Model file for the job. Use its own axes, mm. Give positions to 0.01 mm unless a question says otherwise; leave off trailing zeros. Write each loop counter-clockwise with the first axis right and the second up, starting at its lowest first coordinate (ties: lowest second). Pieces come first, ordered by that corner, then holes. Notation, with made-up numbers: M 64,-2 L 95,-2 A27 cw 95,32 Z; hole C -21.5,53 d9. An arc over 180 degrees is marked long. Answer as a JSON object with one key per item and string values. Group by question number.
```python
from build123d import *

# Parameters (mm, degrees)
BOSS_EXTRUDE1_DEPTH = 10
CUT_EXTRUDE1_REACH  = 12
SKETCH2_R           = 1.5
CUT_EXTRUDE2_REACH  = 12
SKETCH3_R           = 1.3
SKETCH3_R_2         = 7.5


with BuildPart() as part:
    # Sketch1 → Boss-Extrude1 (new body)
    with BuildSketch(Plane.XY):
        with BuildLine():
            Line((-21, 100), (-29.51790497, 5.356611447))
            ThreePointArc((-29.51790497, 5.356611447), (0, 30), (29.51790497, 5.356611447))
            Line((29.51790497, 5.356611447), (21, 100))
            Line((21, 100), (-21, 100))
        make_face()
        with BuildLine():
            Line((-29.51790497, 5.356611447), (-30, 0))
            ThreePointArc((-30, 0), (0, -30), (30, 0))
            Line((30, 0), (29.51790497, 5.356611447))
            ThreePointArc((29.51790497, 5.356611447), (0, 30), (-29.51790497, 5.356611447))
        make_face()
    extrude(amount=BOSS_EXTRUDE1_DEPTH)

    # Sketch2 → Cut-Extrude1 (cut, up to next)
    with BuildSketch(Plane(origin=(0, 0, 0), x_dir=(-1, 0, 0), z_dir=(0, 0, -1)), mode=Mode.PRIVATE) as cut_extrude1_sk1:
        with Locations((7, 92)):
            Circle(SKETCH2_R)
    cut_extrude1_tool1 = extrude(cut_extrude1_sk1.sketch, amount=-CUT_EXTRUDE1_REACH, mode=Mode.PRIVATE) & part.part
    add(cut_extrude1_tool1.solids().sort_by_distance((-7, 92, 0))[0], mode=Mode.SUBTRACT)
    # Sketch2 → Cut-Extrude1 (cut, up to next)
    with BuildSketch(Plane(origin=(0, 0, 0), x_dir=(-1, 0, 0), z_dir=(0, 0, -1)), mode=Mode.PRIVATE) as cut_extrude1_sk2:
        with Locations((7, 77)):
            Circle(SKETCH2_R)
    cut_extrude1_tool2 = extrude(cut_extrude1_sk2.sketch, amount=-CUT_EXTRUDE1_REACH, mode=Mode.PRIVATE) & part.part
    add(cut_extrude1_tool2.solids().sort_by_distance((-7, 77, 0))[0], mode=Mode.SUBTRACT)
    # Sketch2 → Cut-Extrude1 (cut, up to next)
    with BuildSketch(Plane(origin=(0, 0, 0), x_dir=(-1, 0, 0), z_dir=(0, 0, -1)), mode=Mode.PRIVATE) as cut_extrude1_sk3:
        with Locations((-7, 77)):
            Circle(SKETCH2_R)
    cut_extrude1_tool3 = extrude(cut_extrude1_sk3.sketch, amount=-CUT_EXTRUDE1_REACH, mode=Mode.PRIVATE) & part.part
    add(cut_extrude1_tool3.solids().sort_by_distance((7, 77, 0))[0], mode=Mode.SUBTRACT)
    # Sketch2 → Cut-Extrude1 (cut, up to next)
    with BuildSketch(Plane(origin=(0, 0, 0), x_dir=(-1, 0, 0), z_dir=(0, 0, -1)), mode=Mode.PRIVATE) as cut_extrude1_sk4:
        with Locations((-7, 92)):
            Circle(SKETCH2_R)
    cut_extrude1_tool4 = extrude(cut_extrude1_sk4.sketch, amount=-CUT_EXTRUDE1_REACH, mode=Mode.PRIVATE) & part.part
    add(cut_extrude1_tool4.solids().sort_by_distance((7, 92, 0))[0], mode=Mode.SUBTRACT)

    # Sketch3 → Cut-Extrude2 (cut, up to next)
    with BuildSketch(Plane(origin=(0, 0, 0), x_dir=(-1, 0, 0), z_dir=(0, 0, -1)), mode=Mode.PRIVATE) as cut_extrude2_sk1:
        with Locations((0, 13)):
            Circle(SKETCH3_R)
    cut_extrude2_tool1 = extrude(cut_extrude2_sk1.sketch, amount=-CUT_EXTRUDE2_REACH, mode=Mode.PRIVATE) & part.part
    add(cut_extrude2_tool1.solids().sort_by_distance((0, 13, 0))[0], mode=Mode.SUBTRACT)
    # Sketch3 → Cut-Extrude2 (cut, up to next)
    with BuildSketch(Plane(origin=(0, 0, 0), x_dir=(-1, 0, 0), z_dir=(0, 0, -1)), mode=Mode.PRIVATE) as cut_extrude2_sk2:
        with Locations((13, 0)):
            Circle(SKETCH3_R)
    cut_extrude2_tool2 = extrude(cut_extrude2_sk2.sketch, amount=-CUT_EXTRUDE2_REACH, mode=Mode.PRIVATE) & part.part
    add(cut_extrude2_tool2.solids().sort_by_distance((-13, 0, 0))[0], mode=Mode.SUBTRACT)
    # Sketch3 → Cut-Extrude2 (cut, up to next)
    with BuildSketch(Plane(origin=(0, 0, 0), x_dir=(-1, 0, 0), z_dir=(0, 0, -1)), mode=Mode.PRIVATE) as cut_extrude2_sk3:
        with Locations((0, -13)):
            Circle(SKETCH3_R)
    cut_extrude2_tool3 = extrude(cut_extrude2_sk3.sketch, amount=-CUT_EXTRUDE2_REACH, mode=Mode.PRIVATE) & part.part
    add(cut_extrude2_tool3.solids().sort_by_distance((0, -13, 0))[0], mode=Mode.SUBTRACT)
    # Sketch3 → Cut-Extrude2 (cut, up to next)
    with BuildSketch(Plane(origin=(0, 0, 0), x_dir=(-1, 0, 0), z_dir=(0, 0, -1)), mode=Mode.PRIVATE) as cut_extrude2_sk4:
        with Locations((-13, 0)):
            Circle(SKETCH3_R)
    cut_extrude2_tool4 = extrude(cut_extrude2_sk4.sketch, amount=-CUT_EXTRUDE2_REACH, mode=Mode.PRIVATE) & part.part
    add(cut_extrude2_tool4.solids().sort_by_distance((13, 0, 0))[0], mode=Mode.SUBTRACT)
    # Sketch3 → Cut-Extrude2 (cut, up to next)
    with BuildSketch(Plane(origin=(0, 0, 0), x_dir=(-1, 0, 0), z_dir=(0, 0, -1)), mode=Mode.PRIVATE) as cut_extrude2_sk5:
        Circle(SKETCH3_R_2)
    cut_extrude2_tool5 = extrude(cut_extrude2_sk5.sketch, amount=-CUT_EXTRUDE2_REACH, mode=Mode.PRIVATE) & part.part
    add(cut_extrude2_tool5.solids().sort_by_distance((0, 0, 0))[0], mode=Mode.SUBTRACT)


solid = part.part
```
Q1. Wall check: L1, parallel to Y at x = 0, z = 5.5; L2, parallel to X at y = 76, z = 1.75; L3, parallel to Y at x = -8, z = 6. Give the ranges that are in metal, low to high.
Q2. Slice it at C-C, the plane z = 7. Count the separate pieces of the cut face and the enclosed holes in it, then the cut area to 3 significant figures.
Q3. Slice it at D-D, the plane x = 13. Write the cut outline in (y, z), then the cut area to 3 significant figures.
Q4. Two-plate mould, pull along X, no slides. Class faces 1 (the cylindrical face through (-0.66, -29.993, 4.93)), 2 (the flat face through (0, 36, 0)), 3 (the cylindrical face through (0.17, -11.71, 4.93)): +X half, -X half, draft (parallel to the pull), parting line (faces both ways), or undercut.
Q5. Slice it at B-B, the plane x = 0. Write the cut outline in (y, z), then the cut area to 3 significant figures.
Q6. Drop flat-ended pins along their axis: P1, Ø4, axis at y = 82, z = 9, coming from the +X side; P2, Ø4, axis at x = 21.5, z = 2, coming from the -Y side; P3, Ø5, axis at y = 55, z = 2.5, coming from the -X side (3 decimals). Give the stop position or say it passes through.
Q7. Slice it at A-A, the plane y = 92. Write the cut outline in (x, z).
Solved:
{
 "1": {"L1": "y = -30 to -14.3, -11.7 to -7.5, 7.5 to 11.7, 14.3 to 100", "L2": "x = -23.16 to -8.12, -5.88 to 5.88, 8.12 to 23.16", "L3": "y = -28.91 to 75.88, 78.12 to 90.88, 93.12 to 100"},
 "2": {"separate pieces": "1", "enclosed holes": "9", "area": "6,290 mm²"},
 "3": {"outline": "M -27.04,0 L -1.3,0 L -1.3,10 L -27.04,10 Z; M 1.3,0 L 100,0 L 100,10 L 1.3,10 Z", "area": "1,240 mm²"},
 "4": {"face 1": "parting line", "face 2": "draft", "face 3": "undercut"},
 "5": {"outline": "M -30,0 L -14.3,0 L -14.3,10 L -30,10 Z; M -11.7,0 L -7.5,0 L -7.5,10 L -11.7,10 Z; M 7.5,0 L 11.7,0 L 11.7,10 L 7.5,10 Z; M 14.3,0 L 100,0 L 100,10 L 14.3,10 Z", "area": "1,100 mm²"},
 "6": {"P1": "stops at x = 22.8", "P2": "stops at y = -22.8", "P3": "stops at x = -25.275"},
 "7": {"outline": "M -21.72,0 L -8.5,0 L -8.5,10 L -21.72,10 Z; M -5.5,0 L 5.5,0 L 5.5,10 L -5.5,10 Z; M 8.5,0 L 21.72,0 L 21.72,10 L 8.5,10 Z"}
}
